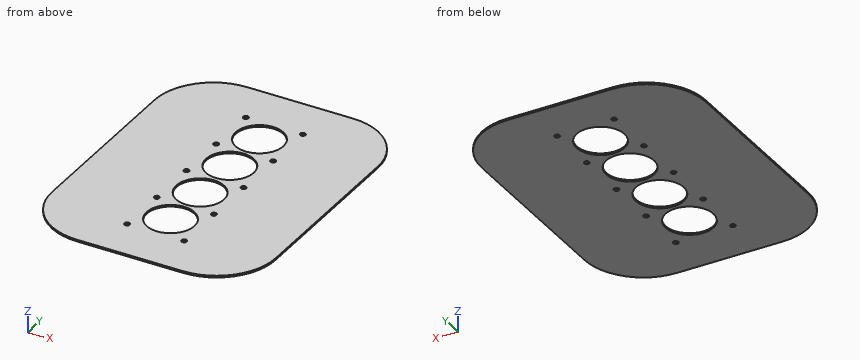
from build123d import *

# Parameters (mm, degrees)
F0_W     = 380
F0_H     = 503
F0_R     = 40.5
F1_DEPTH = 3
F2_R     = 100
F3_D     = 9
F3_DEPTH = 5
F3_TIP   = 2.7038727856


with BuildPart() as f1:
    # F0 (on Top) → F1 (new body)
    with BuildSketch(Plane.XY):
        with Locations((0, -251.5)):
            Rectangle(F0_W, F0_H)
        with Locations((0, -383)):
            Circle(F0_R, mode=Mode.SUBTRACT)
        with Locations((0, -295.5)):
            Circle(F0_R, mode=Mode.SUBTRACT)
        with Locations((0, -207.5)):
            Circle(F0_R, mode=Mode.SUBTRACT)
        with Locations((0, -120)):
            Circle(F0_R, mode=Mode.SUBTRACT)
    extrude(amount=F1_DEPTH)

    # F2
    f2_edges = [f1.edges().sort_by_distance(p)[0] for p in [
        (-190, 0, 1.5),
        (190, 0, 1.5),
        (-190, -503, 1.5),
        (190, -503, 1.5),
    ]]
    fillet(f2_edges, radius=F2_R)

    # F3
    with Locations(Plane(origin=(0, 0, 0), x_dir=(1, 0, 0), z_dir=(0, 0, -1))):
        with Locations((-48.5, 76), (48.5, 76), (-48.5, 163.75), (48.5, 163.75), (-48.5, 251.5), (48.5, 251.5), (-48.5, 339.25), (48.5, 339.25), (-48.5, 427), (48.5, 427)):
            Hole(F3_D / 2, depth=F3_DEPTH)
            with Locations((0, 0, -(F3_DEPTH + F3_TIP / 2))):  # 118° drill point
                Cone(0, F3_D / 2, F3_TIP, mode=Mode.SUBTRACT)


solid = f1.part
CAD build for the part. Positions are in the model's coordinates, mm. Round coordinates to 2 decimals unless told otherwise and drop trailing zeros. Loops run counter-clockwise (first coordinate to the right, second up) from the corner with the lowest first, then second, coordinate; pieces in that order, holes last.
(1) Wall check: line 1 along Y through (x, z) = (48.5, 1); line 2 along Y through (x, z) = (0, 1.3); line 3 along X through (y, z) = (-163.75, 1.7). Give the ranges that are in metal, low to high.
(2) Drop flat-ended pins along their axis: pin 1 (11.5 mm diameter, centred on x = 48.5, y = -339.25, fed in from +Z); pin 2 (1 mm diameter, centred on x = 130.5, z = 2, fed in from +Y). Give the stop position or say it passes through.
(3) Cut at A-A (y = -295.5). Give the cut face in (x, z), plus the area to 3 significant figures.
(4) Cut at C-C (x = 31.5). Give the cut face in (y, z).
(5) Cut at D-D (y = -231.5). Give the cut face in (x, z).
(6) Cut at B-B (z = 2.1). State how many separate pieces and enclosed holes the cut face has, plus the area to 3 significant figures.
Findings below:
1. line 1: y = -503 to -431.5, -422.5 to -343.75, -334.75 to -256, -247 to -168.25, -159.25 to -80.5, -71.5 to 0
1. line 2: y = -503 to -423.5, -342.5 to -336, -255 to -248, -167 to -160.5, -79.5 to 0
1. line 3: x = -190 to -53, -44 to 44, 53 to 190
2. pin 1: stops at z = 3
2. pin 2: stops at y = -8.35
3. outline: (-190, 0) - (-40.5, 0) - (-40.5, 3) - (-190, 3) - close; (40.5, 0) - (190, 0) - (190, 3) - (40.5, 3) - close
3. area: 897 mm2
4. outline: (-503, 0) - (-408.46, 0) - (-408.46, 3) - (-503, 3) - close; (-357.54, 0) - (-320.96, 0) - (-320.96, 3) - (-357.54, 3) - close; (-270.04, 0) - (-232.96, 0) - (-232.96, 3) - (-270.04, 3) - close; (-182.04, 0) - (-145.46, 0) - (-145.46, 3) - (-182.04, 3) - close; (-94.54, 0) - (0, 0) - (0, 3) - (-94.54, 3) - close
5. outline: (-190, 0) - (-32.62, 0) - (-32.62, 3) - (-190, 3) - close; (32.62, 0) - (190, 0) - (190, 3) - (32.62, 3) - close
6. separate pieces: 1
6. enclosed holes: 14
6. area: 161,000 mm2
